Read the model definition and answer for the solid it produces. Units are mm, in the model's axes. Face numbers are marked on the shaded views. A direction names the side the tool comes from. Coordinates: 2 decimals unless noted, no trailing zeros. Order: outer loops, then holes, each group sorted by start corner. A loop starts at its lowest first (then second) coordinate and runs counter-clockwise, first axis right, second up. Notation, with made-up numbers: M -2.75,78.5 L 9.25,78.5 A14 cw 9.25,88.5 Z; hole C 56,-3 d8. An arc over 180 degrees is marked long. One line per question, with ' | ' between items. Start each with the question number.
1) A tool of negligible diameter and unlimited length cuts with its end or side. For the marked faces 1, 2 and 3, from which of +Z, -Z, +X, -X, +Y, -Y can it reach the whole face along a straight path? Write none if from no direction.
2) Consider probe 1 along Y at (x, z) = (26, -106); probe 2 along Y at (x, z) = (-38, -52); probe 3 along X at (y, z) = (24, -12). Determine where each line is inside the solid, lowest interval first.
3) Find section B-B, the plane x = -37.5. Write down the section's boundary in (y, z).
4) Find section A-A, the plane z = -98. Write down the section's boundary in (x, y).
5) Given P1, Ø17.5, axis at y = -9, z = -45, coming from the -X side; P2, Ø4, axis at x = 27.5, y = 17.5, coming from the +Z side; P3, Ø20.5, axis at x = -51, z = -58, coming from the -Y side; P4, Ø9, axis at y = 31.5, z = -63.5, coming from the +X side, each flat-ended and moving along its own axis, determine where each tip first touches the part or whether it passes through.
6) Find section C-C, the plane y = 26.5. Write down the section's boundary in (x, z).
from build123d import *

# Parameters (mm, degrees)
F3_DEPTH = 152.4


# Not quite as in the source:
# - a feature of the source that left no trace in its solid (it failed there, or was rolled back) is left out


with BuildPart() as f3:
    # F2 (on Top) → F3 (new body)
    with BuildSketch(Plane.XY):
        Polygon((-35.4751944542, 0), (-35.4751944542, -34.6453338861), (50.8269667625, -34.6453338861), (50.8269667625, 22.8202939034), (-35.4751944542, 22.8202939034), align=None)
        Polygon((-60.8430989087, 0), (-35.4751944542, 0), (-35.4751944542, 22.8202939034), (-35.4751944542, 34.3115627766), (-60.8430989087, 34.3115627766), align=None)
    extrude(amount=-F3_DEPTH)


solid = f3.part
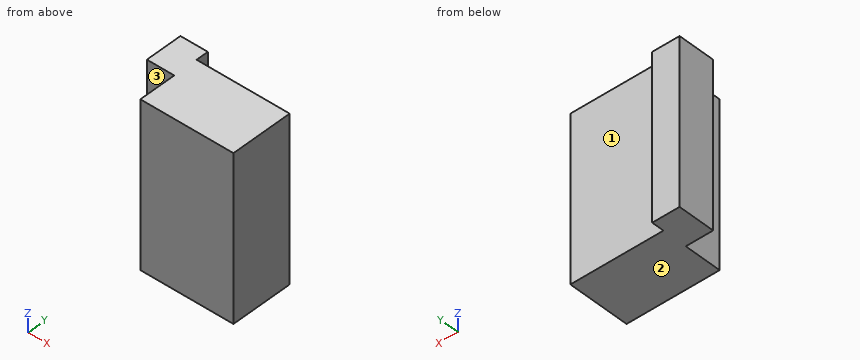
Report:
1) face 1: +Z, -Z, +X, +Y | face 2: -Z, +X, -X, +Y, -Y | face 3: +Z, -Z, -X, -Y
2) probe 1: y = -34.65 to 22.82 | probe 2: y = 0 to 34.31 | probe 3: x = -60.84 to -35.48
3) outline: M 0,-152.4 L 34.31,-152.4 L 34.31,0 L 0,0 Z
4) outline: M -60.84,0 L -35.48,0 L -35.48,-34.65 L 50.83,-34.65 L 50.83,22.82 L -35.48,22.82 L -35.48,34.31 L -60.84,34.31 Z
5) P1: stops at x = -35.48 | P2: stops at z = 0 | P3: stops at y = 0 | P4: stops at x = -35.48
6) outline: M -60.84,-152.4 L -35.48,-152.4 L -35.48,0 L -60.84,0 Z
